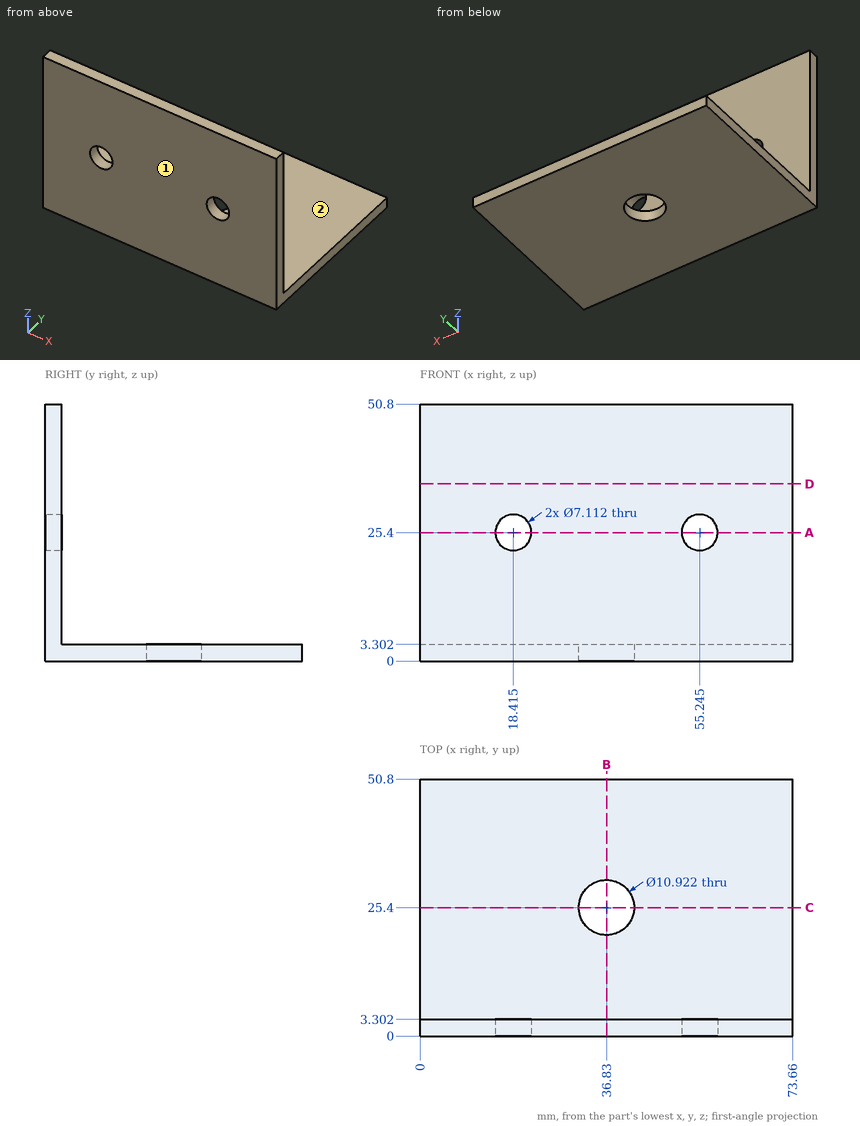
Design review of the part shown in the three views and the two pictorial views. Dimensions are in mm from the part's minimum x, y and z. A direction names the side the tool comes from. Round coordinates to 2 decimals unless told otherwise and drop trailing zeros. Write each loop counter-clockwise with the first axis right and the second up, starting at its lowest first coordinate (ties: lowest second). Pieces come first, ordered by that corner, then holes. Notation, with made-up numbers: (84, -12) - (99, -12) arc R12 ccw to (99, 3) - close; hole circle Ø5 at (17.5, -30). An arc over 180 degrees is marked (long way). Write item = value, one per line. Start each with the question number.
1. Consider section B-B on x = 36.83. State the section outline as (y, z) points, plus the area to 3 significant figures.
2. Consider section A-A on z = 25.4. State the section outline as (x, y) points, plus the area to 3 significant figures.
3. For pin 1 Ø8 at (x, y) = (47, 39) entering from +Z; pin 2 Ø8 at (x, z) = (39.5, 33) entering from -Y; pin 3 Ø1 at (x, z) = (52, 43.5) entering from +Y, all flat-tipped, find the tip position at first contact; note any pin that passes through.
4. Wall thickness on L1, parallel to X at y = 1.85, z = 25.4; L2, parallel to Y at x = 21, z = 10.5: over which ranges is each line inside the solid? List them lowest first.
5. Consider section D-D on z = 35. State the section outline as (x, y) points, plus the area to 3 significant figures.
6. For the marked faces 1 and 2, list the 3-axis set-ups (+Z, -Z, +X, -X, +Y, -Y) from which the entire face can be reached by the end or side of a thin tool; tool diameter is ignored.
7. Consider section C-C on y = 25.4. State the section outline as (x, z) points.
Evaluation:
q1.outline = (0, 0) - (19.94, 0) - (19.94, 3.3) - (3.3, 3.3) - (3.3, 50.8) - (0, 50.8) - close; (30.86, 0) - (50.8, 0) - (50.8, 3.3) - (30.86, 3.3) - close
q1.area = 289 mm2
q2.outline = (0, 0) - (14.86, 0) - (14.86, 3.3) - (0, 3.3) - close; (21.97, 0) - (51.69, 0) - (51.69, 3.3) - (21.97, 3.3) - close; (58.8, 0) - (73.66, 0) - (73.66, 3.3) - (58.8, 3.3) - close
q2.area = 196 mm2
q3.pin_1 = 3.3
q3.pin_2 = 0
q3.pin_3 = 3.3
q4.L1 = 0 to 14.86, 21.97 to 51.69, 58.8 to 73.66
q4.L2 = 0 to 3.3
q5.outline = (0, 0) - (73.66, 0) - (73.66, 3.3) - (0, 3.3) - close
q5.area = 243 mm2
q6.face_1 = +Z, -Z, +X, -X, -Y
q6.face_2 = +Z, +X, -X, +Y
q7.outline = (0, 0) - (31.37, 0) - (31.37, 3.3) - (0, 3.3) - close; (42.29, 0) - (73.66, 0) - (73.66, 3.3) - (42.29, 3.3) - close
